Verification items for the finished model (mm, model axes). A direction names the side the tool comes from. Round coordinates to 2 decimals unless told otherwise and drop trailing zeros. Order: outer loops, then holes, each group sorted by start corner. A loop starts at its lowest first (then second) coordinate and runs counter-clockwise, first axis right, second up. Notation, with made-up numbers: M -20,-40 L 1,-40 A25 cw 1,-21 Z; hole C -3,-1 d7. An arc over 180 degrees is marked long. Use CSV: the item, a comma, the result in double quotes. Start each with the question number.
Q1. Set-up check for faces 5 (the face through (21, -16, 0)), 6 (the face through (-9, 0, 0)), 7 (the face through (0.75, 8, 2)), 8 (the face through (19, -13.4, 0)): record each of +Z, -Z, +X, -X, +Y, -Y from which the full face is reachable in a straight line by a thin tool's end or side.
Q2. Sectioned sample at D-D (z = -5.5). Enter the section's corners in (x, y), and give its area (3 significant figures).
Q3. Mould release check, pull along Z, two halves, no side actions. Record for faces 1 (the face through (-4.426, 7.517, 0.267)), 2 (the face through (-0.75, 8, 2)), 3 (the face through (0, -7, -7)), 4 (the face through (-0.223, -4.669, 6.174)): +Z half, -Z half, draft (parallel to the pull), parting line (faces both ways), or undercut.
Q4. Sectioned sample at A-A (y = 9.55). Enter the section's corners in (x, z).
Q5. Scan lines: line 1 (X direction, y = -15.6, z = 0); line 2 (X direction, y = 6.5, z = -2); line 3 (Y direction, x = -2, z = -0.75). Record each from-to range of solid material in increasing order.
Q6. Gauge pin test, flat ends, axial feed: pin 1 Ø2.5 at (y, z) = (11, -3) entering from +X; pin 2 Ø5.5 at (y, z) = (9.55, 0) entering from +X; pin 3 Ø6 at (y, z) = (11.5, 1) entering from -X. Record the tip position at first contact, or that the pin passes through.
Q7. Sectioned sample at B-B (x = -15). Enter the section's corners in (y, z).
Q8. Sectioned sample at C-C (y = 0.6). Enter the section's corners in (x, z), and give its area (3 significant figures).
Autodesk Inventor part; units mm, degrees
ref_plane "YZ Plane" through (0, 0, 0) normal (1, 0, 0) x (0, 1, 0)
ref_plane "XZ Plane" through (0, 0, 0) normal (0, 1, 0) x (-1, 0, 0)
ref_plane "XY Plane" through (0, 0, 0) normal (0, 0, 1) x (1, 0, 0)
sketch "Эскиз1" plane through (0, 0, 0) normal (0, 0, 1) x (1, 0, 0)
  line L0 (-9, 13.4) -> (9, 13.4)
  line L1 (21, -19.4) -> (-21, -19.4)
  line L2 (-21, -19.4) -> (-21, -13.4)
  line L3 (-9, 13.4) -> (-9, -13.4)
  line L4 (9, 13.4) -> (9, -13.4)
  line L5 (21, -19.4) -> (21, -13.4)
  line L6 (-21, -13.4) -> (-9, -13.4)
  line L7 (9, -13.4) -> (21, -13.4)
  point P0 (0, 0)
  point P1 (-9, 0)
  point P2 (0, -19.4)
  dimension "d0" = 42
  dimension "d2" = 18
  dimension "d3" = 9
  dimension "d6" = 6
  dimension "d7" = 32.8
extrude "Выдавливание1" add sketch "Эскиз1" along normal mid plane 14
sketch "Эскиз3" plane through (0, 0, 7) normal (0, 0, 1) x (1, 0, 0)
  line L0 (-21, -19.4) -> (21, -19.4)
  point P0 (0, 0)
  point P1 (0, 0.6)
  dimension "d12" = 20
hole "Отверстие1" at (0, 0.6, 7) direction (0, 0, -1) diameter 10.2 end through all
sketch "Эскиз4" plane through (0, 0, 7) normal (0, 0, 1) x (1, 0, 0)
  line L0 (-9, 13.4) -> (9, 13.4)
  line L1 (-0.75, 13.4) -> (-0.75, 5.6446)
  circle A0 centre (0, 0.6) radius 5.1
  line L2 (0.75, 13.4) -> (0.75, 5.6446)
  point P0 (0, 0)
  dimension "d20" = 1.5
  dimension "d21" = 0.75
extrude "Выдавливание2" cut sketch "Эскиз4" against normal blind 14 contours L0 L2 A0 L1
sketch "Эскиз6" plane through (9, -13.4, 7) normal (0, 1, 0) x (1, 0, 0)
  line L0 (12, 14) -> (12, 0)
  line L1 (0, 14) -> (12, 14)
  point P0 (-9, 7)
  point P1 (6, 7)
  point P2 (12, 7)
  point P3 (6, 14)
hole "Отверстие3" at (15, -13.4, 0) direction (0, -1, 0) diameter 5.5 end through all
sketch "Эскиз7" plane through (-21, -13.4, 7) normal (0, 1, 0) x (1, 0, 0)
  line L0 (0, 14) -> (12, 14)
  line L1 (0, 0) -> (0, 14)
  point P0 (21, 7)
  point P1 (6, 7)
  point P2 (6, 14)
  point P3 (0, 7)
hole "Отверстие4" at (-15, -13.4, 0) direction (0, -1, 0) diameter 5.5 end through all
sketch "Эскиз8" plane through (9, -13.4, 7) normal (1, 0, 0) x (0, 0, -1)
  line L0 (14, 26.8) -> (0, 26.8)
  point P0 (7, 13.4)
  point P1 (7, 22.95)
  point P2 (7, 26.8)
  dimension "d50" = 3.85
sketch "Эскиз9" plane through (9, -13.4, 7) normal (1, 0, 0) x (0, 0, -1)
  point P0 (7, 13.4)
hole "Отверстие5" at (9, 9.55, 0) direction (-1, 0, 0) diameter 4.1 end through all
thread "Резьба2"
sketch "Эскиз10" plane through (9, -13.4, 7) normal (1, 0, 0) x (0, 0, -1)
  circle A0 centre (7, 22.95) radius 2.5
  line L0 (14, 26.8) -> (0, 26.8)
  point P0 (7, 13.4)
  point P1 (7, 26.8)
  dimension "d60" = 5
  dimension "d61" = 3.85
extrude "Выдавливание3" cut sketch "Эскиз10" against normal blind 5
chamfer "Фаска1" distance 1 angle 45 10 edges at (-5.0861, 0.224, 7) (5.0861, 0.224, 7) (-9, 9.55, 2.05) (-15, -19.4, -2.75) (15, -19.4, -2.75) (-5.0861, 0.224, -7) (5.0861, 0.224, -7) (15, -13.4, -2.75) (-15, -13.4, -2.75) (9, 9.55, 2.5)
properties part number "SK10"
Verdict:
1,face 5,"+Z, -Z, +X, +Y, -Y"
1,face 6,"+Z, -Z, -X, +Y"
1,face 7,"+Z, -Z, +Y"
1,face 8,"+Z, -Z, +X, +Y"
2,outline,"M -21,-19.4 L 21,-19.4 L 21,-13.4 L 9,-13.4 L 9,13.4 L 0.75,13.4 L 0.75,5.64 A5.1 cw long -0.75,5.64 L -0.75,13.4 L -9,13.4 L -9,-13.4 L -21,-13.4 Z"
2,area,"641 mm²"
3,face 1,"undercut"
3,face 2,"draft"
3,face 3,"-Z half"
3,face 4,"+Z half"
4,outline,"M -9,-7 L -0.75,-7 L -0.75,-2.05 L -8,-2.05 L -9,-3.05 Z; M -9,3.05 L -8,2.05 L -0.75,2.05 L -0.75,7 L -9,7 Z; M 0.75,-7 L 9,-7 L 9,-3.5 L 8,-2.5 L 4,-2.5 L 4,-2.05 L 0.75,-2.05 Z; M 0.75,2.05 L 4,2.05 L 4,2.5 L 8,2.5 L 9,3.5 L 9,7 L 0.75,7 Z"
5,line 1,"x = -21 to -17.75, -12.25 to 12.25, 17.75 to 21"
5,line 2,"x = -9 to -0.75, 0.75 to 9"
5,line 3,"y = -19.4 to -4.09, 5.29 to 7.64, 11.46 to 13.4"
6,pin 1,"stops at x = 9"
6,pin 2,"stops at x = 8.25"
6,pin 3,"stops at x = -9"
7,outline,"M -19.4,-7 L -13.4,-7 L -13.4,-3.75 L -14.4,-2.75 L -18.4,-2.75 L -19.4,-3.75 Z; M -19.4,3.75 L -18.4,2.75 L -14.4,2.75 L -13.4,3.75 L -13.4,7 L -19.4,7 Z"
8,outline,"M -9,-7 L -6.1,-7 L -5.1,-6 L -5.1,6 L -6.1,7 L -9,7 Z; M 5.1,-6 L 6.1,-7 L 9,-7 L 9,7 L 6.1,7 L 5.1,6 Z"
8,area,"107 mm²"
